```python
from build123d import *

# Parameters (mm, degrees)
BOSS_EXTRUDE2_DEPTH      = 60
SHELL2_T                 = -7.5
SKETCH14_R               = 4.5
CUT_EXTRUDE3_DEPTH       = 7.5
SKETCH24_W               = 10.2
SKETCH24_H               = 7.5
CUT_EXTRUDE14_DEPTH      = 30
SKETCH20_R               = 1.5
CUT_EXTRUDE15_DEPTH      = 9.9
CUT_EXTRUDE16_REACH      = 87.586
SKETCH20_5_R             = 3.5
CIRPATTERN20_COUNT       = 4
CIRPATTERN21_START       = -24.7500001
CIRPATTERN21_OUTLINE_R   = 3.5
CIRPATTERN21_DEPTH       = 9.7500001
CIRPATTERN21_START_2     = 15
CIRPATTERN21_2_OUTLINE_R = 3.5
CIRPATTERN21_2_DEPTH     = 9.7500001
CIRPATTERN21_START_3     = -15
CIRPATTERN21_3_OUTLINE_R = 1.5
CIRPATTERN21_3_DEPTH     = 30
CIRPATTERN21_4_OUTLINE_R = 3.5
CIRPATTERN21_4_DEPTH     = 9.7500001
CIRPATTERN21_5_OUTLINE_R = 3.5
CIRPATTERN21_5_DEPTH     = 9.7500001
CIRPATTERN21_6_OUTLINE_R = 1.5
CIRPATTERN21_6_DEPTH     = 30
FILLET1_R                = 2
CUT_EXTRUDE17_REACH      = 100.615
SKETCH30_R               = 0.752022917
CUT_EXTRUDE19_START      = -10.606601718
CUT_EXTRUDE19_DEPTH      = 10.606601718
CIRPATTERN30_COUNT       = 4
FILLET4_R                = 2.5


# Read off the part's stored shape, not the designer's step: CirPattern21, Cut-Extrude19
with BuildPart() as part:
    # Sketch11 → Boss-Extrude2 (new body)
    with BuildSketch(Plane(origin=(0, 0, 0), x_dir=(1, 0, 0), z_dir=(0, 1, 0))):
        Polygon((17.5, 35), (0, 35), (-17.5, 35), (-35, 17.5), (-35, 0), (-35, -17.5), (-17.5, -35), (0, -35), (17.5, -35), (35, -17.5), (35, 0), (35, 17.5), align=None)
    extrude(amount=BOSS_EXTRUDE2_DEPTH)

    # Shell2
    shell2_openings = [part.faces().sort_by_distance(p)[0] for p in [
        (0, 0, 0),
    ]]
    offset(amount=SHELL2_T, openings=shell2_openings, kind=Kind.INTERSECTION)

    # Sketch14 → Cut-Extrude3 (cut)
    with BuildSketch(Plane(origin=(0, 60, 0), x_dir=(1, 0, 0), z_dir=(0, 1, 0))):
        with Locations(Location((0, 0, 0), (0, 0, 270))):
            Circle(SKETCH14_R)
    extrude(amount=-CUT_EXTRUDE3_DEPTH, mode=Mode.SUBTRACT)

    # Sketch24 → Cut-Extrude14 (cut)
    with BuildSketch(Plane.XZ):
        with Locations((0, 31.25)):
            Rectangle(SKETCH24_W, SKETCH24_H)
    cut_extrude14 = extrude(amount=-CUT_EXTRUDE14_DEPTH, mode=Mode.SUBTRACT)

    # Sketch20 → Cut-Extrude15 (cut)
    with BuildSketch(Plane(origin=(15, 0, 0), x_dir=(0, 0, -1), z_dir=(1, 0, 0))):
        with Locations((-31.25, 26)):
            Circle(SKETCH20_R)
    cut_extrude15 = extrude(amount=-CUT_EXTRUDE15_DEPTH, mode=Mode.SUBTRACT)

    # Cut-Extrude16: up to this plane
    cut_extrude16_end = Plane(origin=(26.25, 60, 26.25), z_dir=(-0.7071067811864445, 0, -0.7071067811866506))
    # Sketch20<5> → Cut-Extrude16 (cut, up to the surface)
    with BuildSketch(Plane(origin=(15, 0, 0), x_dir=(0, 0, -1), z_dir=(1, 0, 0)), mode=Mode.PRIVATE) as cut_extrude16_sk1:
        with Locations(Location((-31.25, 26, 0), (0, 0, 180))):
            Circle(SKETCH20_5_R)
    cut_extrude16_tool1 = split(extrude(cut_extrude16_sk1.sketch, amount=CUT_EXTRUDE16_REACH, mode=Mode.PRIVATE), bisect_by=cut_extrude16_end, keep=Keep.BOTH, mode=Mode.PRIVATE)
    cut_extrude16 = cut_extrude16_tool1.solids().sort_by_distance((15, 26, 31.25))[0]
    add(cut_extrude16, mode=Mode.SUBTRACT)

    # Mirror2: Cut-Extrude15, Cut-Extrude16 across plane
    add(cut_extrude15.mirror(Plane(origin=(0, 0, 0), x_dir=(0, 0, 1), z_dir=(1, 0, 0))), mode=Mode.SUBTRACT)
    add(cut_extrude16.mirror(Plane(origin=(0, 0, 0), x_dir=(0, 0, 1), z_dir=(1, 0, 0))), mode=Mode.SUBTRACT)

    # CirPattern20: Cut-Extrude14 ×4 about axis
    cirpattern20_axis = Axis((0, 0, 0), (0, 1, 0))
    for i in range(1, CIRPATTERN20_COUNT):
        add(cut_extrude14.rotate(cirpattern20_axis, i * 360 / CIRPATTERN20_COUNT), mode=Mode.SUBTRACT)

    # CirPattern21 outline → CirPattern21 (cut)
    with BuildSketch(Plane.YZ.offset(CIRPATTERN21_START)):
        with Locations((26, -31.25)):
            Circle(CIRPATTERN21_OUTLINE_R)
    extrude(amount=CIRPATTERN21_DEPTH, mode=Mode.SUBTRACT)

    # CirPattern21 2 outline → CirPattern21 2 (cut)
    with BuildSketch(Plane.YZ.offset(CIRPATTERN21_START_2)):
        with Locations((26, -31.25)):
            Circle(CIRPATTERN21_2_OUTLINE_R)
    extrude(amount=CIRPATTERN21_2_DEPTH, mode=Mode.SUBTRACT)

    # CirPattern21 3 outline → CirPattern21 3 (cut)
    with BuildSketch(Plane.YZ.offset(CIRPATTERN21_START_3)):
        with Locations((26, -31.25)):
            Circle(CIRPATTERN21_3_OUTLINE_R)
    extrude(amount=CIRPATTERN21_3_DEPTH, mode=Mode.SUBTRACT)

    # CirPattern21 4 outline → CirPattern21 4 (cut)
    with BuildSketch(Plane.XY.offset(CIRPATTERN21_START)):
        with Locations((-31.25, 26)):
            Circle(CIRPATTERN21_4_OUTLINE_R)
        with Locations((31.25, 26)):
            Circle(CIRPATTERN21_4_OUTLINE_R)
    extrude(amount=CIRPATTERN21_4_DEPTH, mode=Mode.SUBTRACT)

    # CirPattern21 5 outline → CirPattern21 5 (cut)
    with BuildSketch(Plane.XY.offset(CIRPATTERN21_START_2)):
        with Locations((-31.25, 26)):
            Circle(CIRPATTERN21_5_OUTLINE_R)
        with Locations((31.25, 26)):
            Circle(CIRPATTERN21_5_OUTLINE_R)
    extrude(amount=CIRPATTERN21_5_DEPTH, mode=Mode.SUBTRACT)

    # CirPattern21 6 outline → CirPattern21 6 (cut)
    with BuildSketch(Plane.XY.offset(CIRPATTERN21_START_3)):
        with Locations((-31.25, 26)):
            Circle(CIRPATTERN21_6_OUTLINE_R)
        with Locations((31.25, 26)):
            Circle(CIRPATTERN21_6_OUTLINE_R)
    extrude(amount=CIRPATTERN21_6_DEPTH, mode=Mode.SUBTRACT)

    # Fillet1
    fillet1_edges = [part.edges().sort_by_distance(p)[0] for p in [
        (-27.5, 30, 0),
        (-35, 30, 0),
        (0, 30, -27.5),
        (0, 30, -35),
        (27.5, 30, 0),
        (35, 30, 0),
        (0, 30, 27.5),
        (0, 30, 35),
    ]]
    fillet(fillet1_edges, radius=FILLET1_R)

    # Sketch30 → Cut-Extrude17 (cut, up to next)
    with BuildSketch(Plane.XY.offset(35), mode=Mode.PRIVATE) as cut_extrude17_sk1:
        with Locations((2.5, 36.5)):
            Circle(SKETCH30_R)
    cut_extrude17_tool1 = extrude(cut_extrude17_sk1.sketch, amount=-CUT_EXTRUDE17_REACH, mode=Mode.PRIVATE) & part.part
    # Sketch30 → Cut-Extrude17 (cut, up to next)
    with BuildSketch(Plane.XY.offset(35), mode=Mode.PRIVATE) as cut_extrude17_sk2:
        with Locations(Location((-2.5, 36.5, 0), (0, 0, 180))):
            Circle(SKETCH30_R)
    cut_extrude17_tool2 = extrude(cut_extrude17_sk2.sketch, amount=-CUT_EXTRUDE17_REACH, mode=Mode.PRIVATE) & part.part
    cut_extrude17_1 = cut_extrude17_tool1.solids().sort_by_distance((2.5, 36.5, 35))[0]
    add(cut_extrude17_1, mode=Mode.SUBTRACT)
    cut_extrude17_2 = cut_extrude17_tool2.solids().sort_by_distance((-2.5, 36.5, 35))[0]
    add(cut_extrude17_2, mode=Mode.SUBTRACT)
    cut_extrude17 = cut_extrude17_1 + cut_extrude17_2  # Cut-Extrude17 as one shape, for the pattern or mirror that repeats it

    # Cut-Extrude19 outline → Cut-Extrude19 (cut)
    with BuildSketch(Plane(origin=(35, 0, 0), x_dir=(0, 0, -1), z_dir=(1, 0, 0)).offset(CUT_EXTRUDE19_START)):
        Polygon((17.5, 0), (14.5, 15), (5.1, 15), (5.1, 0), align=None)
        Polygon((-5.1, 0), (-5.1, 15), (-14.5, 15), (-17.5, 0), align=None)
    cut_extrude19 = extrude(amount=CUT_EXTRUDE19_DEPTH, mode=Mode.SUBTRACT)

    # CirPattern30: Cut-Extrude17, Cut-Extrude19 ×4 about axis
    cirpattern30_axis = Axis((0, 0, 0), (0, 1, 0))
    add([cut_extrude17.rotate(cirpattern30_axis, i * 360 / CIRPATTERN30_COUNT) for i in range(1, CIRPATTERN30_COUNT)], mode=Mode.SUBTRACT)
    add([cut_extrude19.rotate(cirpattern30_axis, i * 360 / CIRPATTERN30_COUNT) for i in range(1, CIRPATTERN30_COUNT)], mode=Mode.SUBTRACT)

    # Fillet4
    fillet4_edges = [part.edges().sort_by_distance(p)[0] for p in [
        (31.196699141, 15, -14.5),
        (31.196699141, 15, 14.5),
        (14.5, 15, -31.196699141),
        (-14.5, 15, -31.196699141),
        (-31.196699141, 15, -14.5),
        (-31.196699141, 15, 14.5),
        (-14.5, 15, 31.196699141),
        (14.5, 15, 31.196699141),
    ]]
    fillet(fillet4_edges, radius=FILLET4_R)


solid = part.part
```
Model file for the job. Use its own axes, mm. A direction names the side the tool comes from. Give positions to 0.01 mm unless a question says otherwise; leave off trailing zeros. Write each loop counter-clockwise with the first axis right and the second up, starting at its lowest first coordinate (ties: lowest second). Pieces come first, ordered by that corner, then holes. Notation, with made-up numbers: (12.25, 32) - (35.25, 32) arc R14 ccw to (35.25, 41) - close; hole circle Ø11 at (-16, -18). An arc over 180 degrees is marked (long way). One line per question, with ' | ' between items. Start each with the question number.
(1) Slice it at D-D on z = 0. Write the cut outline in (x, y).
(2) Slice it at A-A on x = -31.25. Give the number of separate pieces and of enclosed holes in the cut face, plus the area to 3 significant figures.
(3) Pin check, flat tips, straight feed: P1, Ø1.8, axis at x = 31, z = -0.5, coming from the -Y side; P2, Ø5.5, axis at y = 26.5, z = -31.5, coming from the +X side; P3, Ø11, axis at y = 26, z = -31.25, coming from the +X side; P4, Ø2.5, axis at y = 26, z = -31.25, coming from the -X side. Stop position of each tip, or through.
(4) 3-axis set-ups, long thin cutter, end or side, ignore diameter. For faces 1 (the face through (-16.18, 6.59, 30.8)), 2 (the face through (30.8, 6.59, 16.18)), 3 (the face through (-34.43, 30.6, 0.07)): which of +Z, -Z, +X, -X, +Y, -Y reach the whole face in a straight line?
(5) Wall check: line 1 along X through (y, z) = (26, 12.5); line 2 along X through (y, z) = (55, 0); line 3 along X through (y, z) = (35.5, -11.5). Give the ranges that are in metal, low to high. Write a range as from..to.
(6) Two-plate mould, pull along Y, no slides. Class faces 4 (the face through (24, 0, -24)), 5 (the face through (-31, 21, -5.1)), 6 (the face through (30.14, 27.01, 9.98)): +Y half, -Y half, draft (parallel to the pull), parting line (faces both ways), or undercut.
(7) Slice it at B-B on x = 0. Write the cut outline in (y, z).
Results below:
1) outline: (-35, 32) arc R2 ccw to (-33, 30) - (-29.5, 30) arc R2 ccw to (-27.5, 32) - (-27.5, 52.5) - (-4.5, 52.5) - (-4.5, 60) - (-35, 60) - close; (4.5, 52.5) - (27.5, 52.5) - (27.5, 32) arc R2 ccw to (29.5, 30) - (33, 30) arc R2 ccw to (35, 32) - (35, 60) - (4.5, 60) - close
2) separate pieces: 3 | enclosed holes: 2 | area: 1,770 mm^2
3) P1: y = 30 | P2: x = 15 | P3: x = 26.75 | P4: through
4) face 1: +Z, -Z, -Y | face 2: +X, -X, -Y | face 3: -X, -Y
5) line 1: -35..-32.75, -29.75..-27.5, 27.5..29.75, 32.75..35 | line 2: -35..-4.5, 4.5..35 | line 3: -35..-27.5, 27.5..35
6) face 4: -Y half | face 5: draft | face 6: undercut
7) outline: (30, -33) arc R2 ccw to (32, -35) - (60, -35) - (60, -4.5) - (52.5, -4.5) - (52.5, -27.5) - (32, -27.5) arc R2 ccw to (30, -29.5) - close; (30, 29.5) arc R2 ccw to (32, 27.5) - (52.5, 27.5) - (52.5, 4.5) - (60, 4.5) - (60, 35) - (32, 35) arc R2 ccw to (30, 33) - close
